from build123d import *

# Parameters (mm, degrees)
F0_W     = 112
F0_H     = 76
F1_DEPTH = 12
F4_DEPTH = 56
F5_W     = 46.2375640869
F5_H     = 25
F6_DEPTH = 40


with BuildPart() as f1:
    # F0 (on Front) → F1 (new body)
    with BuildSketch(Plane.XZ):
        Rectangle(F0_W, F0_H)
    extrude(amount=F1_DEPTH)

    # F3 (on offset) → F4 (join)
    with BuildSketch(Plane(origin=(0, 0, -28), x_dir=(1, 0, 0), z_dir=(0, 0, -1))):
        Polygon((-25, 62), (-56, 12), (56, 12), (25, 62), align=None)
    extrude(amount=-F4_DEPTH)

    # F5 (on face) → F6 (cut)
    with BuildSketch(Plane.XZ.offset(62)):
        Polygon((-33.4565163767, -12.5), (-25, -12.5), (-25, 12.5), (-33.4565163767, 12.5), (-89.381583035, 12.5), (-89.381583035, -12.5), align=None)
        with Locations((48.1187820435, 0)):
            Rectangle(F5_W, F5_H)
        Polygon((-25, -12.5), (24.235787726, -12.5), (25, -12.5), (25, 12.5), (24.235787726, 12.5), (-25, 12.5), align=None)
    extrude(amount=-F6_DEPTH, mode=Mode.SUBTRACT)


solid = f1.part
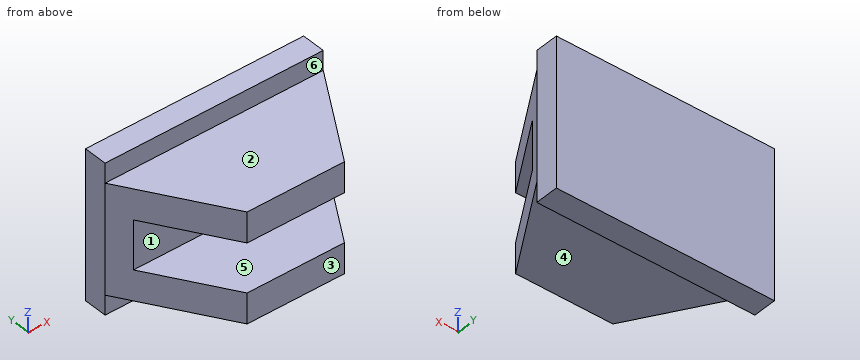
Geometry check sheet. Reference: the model listing, model coordinates, mm. Face numbers are marked on the shaded views. A direction names the side the tool comes from. Round coordinates to 2 decimals unless told otherwise and drop trailing zeros. Order: outer loops, then holes, each group sorted by start corner. A loop starts at its lowest first (then second) coordinate and runs counter-clockwise, first axis right, second up. Notation, with made-up numbers: M 28.25,-3 L 56.25,-3 A28 ccw 56.25,15 Z; hole C 37.5,69 d10. An arc over 180 degrees is marked long. Answer in a Markdown table with one row per item. Add a question column.
Item 1: Set-up check for the marked faces 1, 2 and 3: record each of +Z, -Z, +X, -X, +Y, -Y from which the full face is reachable in a straight line by a thin tool's end or side.
Item 2: Sectioned sample at D-D, the plane z = -18. Enter the section's corners in (x, y).
Item 3: Sectioned sample at C-C, the plane x = -8.5. Enter the section's corners in (y, z).
Item 4: Material ranges on L1, parallel to Z at x = 32, y = -41.5; L2, parallel to Y at x = -34, z = -9; L3, parallel to Y at x = -33.5, z = -31.5, recorded low to high. Write a range as [from, to].
Item 5: Depth check by flat-ended pin: pin 1 Ø8 at (x, y) = (-19, -38.5) entering from -Z; pin 2 Ø6 at (y, z) = (-28.5, 18) entering from -X; pin 3 Ø25 at (x, y) = (12.5, -28.5) entering from +Z. Enter the tip coordinate at first touch or a pass-through.
Item 6: Draft check along Z on the marked faces 4, 5 and 6. Enter one of: released by +Z, released by -Z, zero draft, split by the parting line, or undercut.
Item 7: Sectioned sample at B-B, the plane y = -41.5. Enter the section's corners in (x, z).
Item 8: Sectioned sample at A-A, the plane y = -52.5. Enter the section's corners in (x, z).
Filled in:
| question | item | result |
|---|---|---|
| 1 | face 1 | +X, -X, -Y |
| 1 | face 2 | +Z, +X, -X, -Y |
| 1 | face 3 | +Z, -Z, +X, -X, -Y |
| 2 | outline | M -56,-12 L -25,-62 L 25,-62 L 56,-12 L 56,0 L -56,0 Z |
| 3 | outline | M -62,-28 L -12,-28 L -12,-38 L 0,-38 L 0,38 L -12,38 L -12,28 L -62,28 L -62,12.5 L -22,12.5 L -22,-12.5 L -62,-12.5 Z |
| 4 | L1 | z = [-28, -12.5], [12.5, 28] |
| 4 | L2 | y = [-22, 0] |
| 4 | L3 | y = [-12, 0] |
| 5 | pin 1 | stops at z = -28 |
| 5 | pin 2 | stops at x = -47.63 |
| 5 | pin 3 | stops at z = 28 |
| 6 | face 4 | released by -Z |
| 6 | face 5 | undercut |
| 6 | face 6 | zero draft |
| 7 | outline | M -37.71,-28 L 37.71,-28 L 37.71,-12.5 L -37.71,-12.5 Z; M -37.71,12.5 L 37.71,12.5 L 37.71,28 L -37.71,28 Z |
| 8 | outline | M -30.89,-28 L 30.89,-28 L 30.89,-12.5 L -30.89,-12.5 Z; M -30.89,12.5 L 30.89,12.5 L 30.89,28 L -30.89,28 Z |
